from build123d import *

# Parameters (mm, degrees)
SKETCH2_W           = 35.052
SKETCH2_H           = 79.375
BOSS_EXTRUDE1_DEPTH = 22.225
SKETCH3_R           = 1.5875
BOSS_EXTRUDE2_DEPTH = 3.175
BOSS_EXTRUDE4_DEPTH = 22.225
FILLET2_R           = 3.175
BOSS_EXTRUDE5_DEPTH = 0.00254
BOSS_EXTRUDE6_START = 0.00254
BOSS_EXTRUDE6_DEPTH = 0.00254
BOSS_EXTRUDE7_DEPTH = 6.35
SKETCH8_R           = 7.441189758
SKETCH8_R_2         = 3.175
CUT_EXTRUDE2_DEPTH  = 1.5875
FILLET3_R           = 1.5875
FILLET5_R           = 1.5875
SKETCH9_R           = 4.1275
CUT_EXTRUDE3_DEPTH  = 6.858
SKETCH10_R          = 4.1275
CUT_EXTRUDE4_DEPTH  = 6.858
SKETCH11_R          = 1.5875
CUT_EXTRUDE5_DEPTH  = 91.861200127


with BuildPart() as part:
    # Sketch2 → Boss-Extrude1 (new body)
    with BuildSketch(Plane.XY):
        with Locations((17.526, 39.6875)):
            Rectangle(SKETCH2_W, SKETCH2_H)
    extrude(amount=BOSS_EXTRUDE1_DEPTH)

    # Sketch3 → Boss-Extrude2 (add)
    with BuildSketch(Plane(origin=(35.052, 0, 0), x_dir=(0, 0, -1), z_dir=(1, 0, 0))):
        with Locations(Location((-11.1125, 6.985, 0), (0, 0, 180))):
            Circle(SKETCH3_R)
    extrude(amount=BOSS_EXTRUDE2_DEPTH)

    # Sketch4 → Boss-Extrude4 (add)
    with BuildSketch(Plane.XY.offset(22.225)):
        Polygon((30.48, -3.81), (30.48, 0), (29.21, 0), (3.81, 0), (3.81, -29.21), (35.052, -29.21), (35.052, -9.836099718), align=None)
    extrude(amount=-BOSS_EXTRUDE4_DEPTH)

    # Fillet2
    fillet2_edges = [part.edges().sort_by_distance(p)[0] for p in [
        (30.48, -3.81, 11.1125),
        (35.052, -9.836099718, 11.1125),
        (35.052, -29.21, 11.1125),
        (3.81, -29.21, 11.1125),
    ]]
    fillet(fillet2_edges, radius=FILLET2_R)

    # Sketch5 → Boss-Extrude5 (add)
    with BuildSketch(Plane.XY.offset(22.225)):
        with BuildLine():
            Line((3.81, 0), (30.48, 0))
            Line((30.48, 0), (30.48, -2.741877551))
            ThreePointArc((30.48, -2.741877551), (30.64572555, -3.754247187), (31.125601437, -4.660931461))
            Line((31.125601437, -4.660931461), (34.406398563, -8.985168257))
            ThreePointArc((34.406398563, -8.985168257), (34.88627445, -9.891852531), (35.052, -10.904222168))
            Line((35.052, -10.904222168), (35.052, -26.035))
            ThreePointArc((35.052, -26.035), (34.12206403, -28.28006403), (31.877, -29.21))
            Line((31.877, -29.21), (6.985, -29.21))
            ThreePointArc((6.985, -29.21), (4.73993597, -28.28006403), (3.81, -26.035))
            Line((3.81, -26.035), (3.81, 0))
        make_face()
    extrude(amount=BOSS_EXTRUDE5_DEPTH)

    # Sketch6 → Boss-Extrude6 (add)
    with BuildSketch(Plane(origin=(0, 0, 0), x_dir=(-1, 0, 0), z_dir=(0, 0, -1)).offset(BOSS_EXTRUDE6_START)):
        with BuildLine():
            Line((-30.48, 0), (-3.81, 0))
            Line((-3.81, 0), (-3.81, -26.035))
            ThreePointArc((-3.81, -26.035), (-4.73993597, -28.28006403), (-6.985, -29.21))
            Line((-6.985, -29.21), (-31.877, -29.21))
            ThreePointArc((-31.877, -29.21), (-34.12206403, -28.28006403), (-35.052, -26.035))
            Line((-35.052, -26.035), (-35.052, -10.904222168))
            ThreePointArc((-35.052, -10.904222168), (-34.88627445, -9.891852531), (-34.406398563, -8.985168257))
            Line((-34.406398563, -8.985168257), (-31.125601437, -4.660931461))
            ThreePointArc((-31.125601437, -4.660931461), (-30.64572555, -3.754247187), (-30.48, -2.741877551))
            Line((-30.48, -2.741877551), (-30.48, 0))
        make_face()
    extrude(amount=-BOSS_EXTRUDE6_DEPTH)

    # Sketch7 → Boss-Extrude7 (add)
    with BuildSketch(Plane.XZ.offset(29.21)):
        Polygon((17.890627537, 15.85327897), (15.398252537, 14.042462536), (14.44625, 11.1125), (15.398252537, 8.182537464), (17.890627537, 6.37172103), (20.971372463, 6.37172103), (23.463747463, 8.182537464), (24.41575, 11.1125), (23.463747463, 14.042462536), (20.971372463, 15.85327897), align=None)
    extrude(amount=BOSS_EXTRUDE7_DEPTH)

    # Sketch8 → Cut-Extrude2 (cut)
    # profile 1 of 2: a face of its own
    with BuildSketch(Plane.XZ.offset(29.21)):
        with Locations((19.431, 11.1125)):
            Circle(SKETCH8_R)
        Polygon((14.44625, 11.1125), (15.398252537, 14.042462536), (17.890627537, 15.85327897), (20.971372463, 15.85327897), (23.463747463, 14.042462536), (24.41575, 11.1125), (23.463747463, 8.182537464), (20.971372463, 6.37172103), (17.890627537, 6.37172103), (15.398252537, 8.182537464), align=None, mode=Mode.SUBTRACT)
    # profile 2 of 2: a face of its own
    with BuildSketch(Plane.XZ.offset(29.21)):
        Polygon((15.398252537, 14.042462536), (17.890627537, 15.85327897), (20.971372463, 15.85327897), (23.463747463, 14.042462536), (24.41575, 11.1125), (23.463747463, 8.182537464), (20.971372463, 6.37172103), (17.890627537, 6.37172103), (15.398252537, 8.182537464), (14.44625, 11.1125), align=None)
        with Locations(Location((19.431, 11.1125, 0), (0, 0, 270))):
            Circle(SKETCH8_R_2, mode=Mode.SUBTRACT)
    extrude(amount=CUT_EXTRUDE2_DEPTH, mode=Mode.SUBTRACT)

    # Fillet3
    fillet3_edges = [part.edges().sort_by_distance(p)[0] for p in [
        (0, 79.375, 11.1125),
        (35.052, 79.375, 11.1125),
        (35.052, 0, 11.1125),
        (0, 0, 11.1125),
    ]]
    fillet(fillet3_edges, radius=FILLET3_R)

    # Fillet5
    # the kernel refuses this fillet: 1.5875 mm, written as the material it takes off along each edge
    with BuildSketch(Plane(origin=(30.48, -2.741877551, -0.00254), x_dir=(0, 0, 1), z_dir=(0, 1, 0)), Plane(origin=(30.48, 0, 22.22754), x_dir=(0, 0, -1), z_dir=(0, -1, 0))) as fillet5_piece_1:
        with BuildLine():
            CenterArc((FILLET5_R, -FILLET5_R), FILLET5_R, 90, 90)
            Line((0, -FILLET5_R), (0, 0))
            Line((0, 0), (FILLET5_R, 0))
        make_face()
    extrude(amount=2.741877551, mode=Mode.SUBTRACT)
    with BuildSketch(Plane(origin=(33.655, -2.741877551, -0.00254), x_dir=(-0.7966609646289196, -0.6044264284729114, 0), z_dir=(0.6044264284729114, -0.7966609646289196, 0))) as fillet5_piece_2:
        with BuildLine():
            CenterArc((3.175 + FILLET5_R, -FILLET5_R), FILLET5_R, 90, 90)
            Line((3.175, -FILLET5_R), (3.175, 0))
            Line((3.175, 0), (3.175 + FILLET5_R, 0))
        make_face()
    revolve(axis=Axis((33.655, -2.741877551, -0.00254), (0, 0, -1)), revolution_arc=37.18757939, mode=Mode.SUBTRACT)
    with BuildSketch(Plane(origin=(34.406398563, -8.985168257, -0.00254), x_dir=(-0.796660964628914, -0.6044264284729185, 0), z_dir=(-0.6044264284729186, 0.7966609646289141, 0)), Plane(origin=(31.125601437, -4.660931461, 22.22754), x_dir=(-0.7966609646289139, -0.6044264284729186, 0), z_dir=(0.6044264284729186, -0.796660964628914, 0))) as fillet5_piece_3:
        with BuildLine():
            CenterArc((FILLET5_R, FILLET5_R), FILLET5_R, 180, 90)
            Line((0, FILLET5_R), (0, 0))
            Line((0, 0), (FILLET5_R, 0))
        make_face()
    extrude(amount=5.427951146, mode=Mode.SUBTRACT)
    with BuildSketch(Plane(origin=(31.877, -10.904222168, -0.00254), x_dir=(1, 0, 0), z_dir=(0, -1, 0))) as fillet5_piece_4:
        with BuildLine():
            CenterArc((3.175 - FILLET5_R, FILLET5_R), FILLET5_R, 270, 90)
            Line((3.175, FILLET5_R), (3.175, 0))
            Line((3.175, 0), (3.175 - FILLET5_R, 0))
        make_face()
    revolve(axis=Axis((31.877, -10.904222168, -0.00254), (0, 0, 1)), revolution_arc=37.18757939, mode=Mode.SUBTRACT)
    with BuildSketch(Plane(origin=(35.052, -26.035, -0.00254), x_dir=(-1, 0, 0), z_dir=(0, 1, 0)), Plane(origin=(35.052, -10.904222168, 22.22754), x_dir=(-1, 0, 0), z_dir=(0, -1, 0))) as fillet5_piece_5:
        with BuildLine():
            CenterArc((FILLET5_R, FILLET5_R), FILLET5_R, 180, 90)
            Line((0, FILLET5_R), (0, 0))
            Line((0, 0), (FILLET5_R, 0))
        make_face()
    extrude(amount=15.130777832, mode=Mode.SUBTRACT)
    with BuildSketch(Plane(origin=(31.877, -26.035, -0.00254), x_dir=(0, -1, 0), z_dir=(-1, 0, 0))) as fillet5_piece_6:
        with BuildLine():
            CenterArc((3.175 - FILLET5_R, FILLET5_R), FILLET5_R, 270, 90)
            Line((3.175, FILLET5_R), (3.175, 0))
            Line((3.175, 0), (3.175 - FILLET5_R, 0))
        make_face()
    revolve(axis=Axis((31.877, -26.035, -0.00254), (0, 0, 1)), revolution_arc=90, mode=Mode.SUBTRACT)
    with BuildSketch(Plane(origin=(6.985, -29.21, -0.00254), x_dir=(0, 1, 0), z_dir=(1, 0, 0)), Plane(origin=(31.877, -29.21, 22.22754), x_dir=(0, 1, 0), z_dir=(-1, 0, 0))) as fillet5_piece_7:
        with BuildLine():
            CenterArc((FILLET5_R, FILLET5_R), FILLET5_R, 180, 90)
            Line((0, FILLET5_R), (0, 0))
            Line((0, 0), (FILLET5_R, 0))
        make_face()
    extrude(amount=24.892, mode=Mode.SUBTRACT)
    with BuildSketch(Plane(origin=(6.985, -26.035, -0.00254), x_dir=(-1, 0, 0), z_dir=(0, 1, 0))) as fillet5_piece_8:
        with BuildLine():
            CenterArc((3.175 - FILLET5_R, FILLET5_R), FILLET5_R, 270, 90)
            Line((3.175, FILLET5_R), (3.175, 0))
            Line((3.175, 0), (3.175 - FILLET5_R, 0))
        make_face()
    revolve(axis=Axis((6.985, -26.035, -0.00254), (0, 0, 1)), revolution_arc=90, mode=Mode.SUBTRACT)
    with BuildSketch(Plane(origin=(3.81, 0, -0.00254), x_dir=(0, 0, 1), z_dir=(0, -1, 0)), Plane(origin=(3.81, -26.035, 22.22754), x_dir=(0, 0, -1), z_dir=(0, 1, 0))) as fillet5_piece_9:
        with BuildLine():
            CenterArc((FILLET5_R, -FILLET5_R), FILLET5_R, 90, 90)
            Line((0, -FILLET5_R), (0, 0))
            Line((0, 0), (FILLET5_R, 0))
        make_face()
    extrude(amount=26.035, mode=Mode.SUBTRACT)
    with BuildSketch(Plane(origin=(6.985, -26.035, 22.22754), x_dir=(0, -1, 0), z_dir=(1, 0, 0))) as fillet5_piece_10:
        with BuildLine():
            CenterArc((3.175 - FILLET5_R, FILLET5_R), FILLET5_R, 270, 90)
            Line((3.175, FILLET5_R), (3.175, 0))
            Line((3.175, 0), (3.175 - FILLET5_R, 0))
        make_face()
    revolve(axis=Axis((6.985, -26.035, 22.22754), (0, 0, -1)), revolution_arc=90, mode=Mode.SUBTRACT)
    with BuildSketch(Plane(origin=(31.877, -26.035, 22.22754), x_dir=(1, 0, 0), z_dir=(0, 1, 0))) as fillet5_piece_11:
        with BuildLine():
            CenterArc((3.175 - FILLET5_R, FILLET5_R), FILLET5_R, 270, 90)
            Line((3.175, FILLET5_R), (3.175, 0))
            Line((3.175, 0), (3.175 - FILLET5_R, 0))
        make_face()
    revolve(axis=Axis((31.877, -26.035, 22.22754), (0, 0, -1)), revolution_arc=90, mode=Mode.SUBTRACT)
    with BuildSketch(Plane(origin=(31.877, -10.904222168, 22.22754), x_dir=(0.7966609646289129, 0.6044264284729202, 0), z_dir=(-0.6044264284729202, 0.7966609646289129, 0))) as fillet5_piece_12:
        with BuildLine():
            CenterArc((3.175 - FILLET5_R, FILLET5_R), FILLET5_R, 270, 90)
            Line((3.175, FILLET5_R), (3.175, 0))
            Line((3.175, 0), (3.175 - FILLET5_R, 0))
        make_face()
    revolve(axis=Axis((31.877, -10.904222168, 22.22754), (0, 0, -1)), revolution_arc=37.18757939, mode=Mode.SUBTRACT)
    with BuildSketch(Plane(origin=(33.655, -2.741877551, 22.22754), x_dir=(-1, 0, 0), z_dir=(0, 1, 0))) as fillet5_piece_13:
        with BuildLine():
            CenterArc((3.175 + FILLET5_R, -FILLET5_R), FILLET5_R, 90, 90)
            Line((3.175, -FILLET5_R), (3.175, 0))
            Line((3.175, 0), (3.175 + FILLET5_R, 0))
        make_face()
    revolve(axis=Axis((33.655, -2.741877551, 22.22754), (0, 0, 1)), revolution_arc=37.18757939, mode=Mode.SUBTRACT)

    # Sketch9 → Cut-Extrude3 (cut)
    with BuildSketch(Plane(origin=(35.052, 0, 0), x_dir=(0, 0, -1), z_dir=(1, 0, 0))):
        with Locations((-11.1125, 55.88)):
            Circle(SKETCH9_R)
        with Locations((-11.1125, 36.83)):
            Circle(SKETCH9_R)
    extrude(amount=-CUT_EXTRUDE3_DEPTH, mode=Mode.SUBTRACT)

    # Sketch10 → Cut-Extrude4 (cut)
    with BuildSketch(Plane.ZY):
        with Locations((11.1125, 65.7225)):
            Circle(SKETCH10_R)
        with Locations((11.1125, 46.6725)):
            Circle(SKETCH10_R)
        with Locations((11.1125, 27.6225)):
            Circle(SKETCH10_R)
    extrude(amount=-CUT_EXTRUDE4_DEPTH, mode=Mode.SUBTRACT)

    # Sketch11 → Cut-Extrude5 (cut, through all)
    with BuildSketch(Plane.XY.offset(22.225)):
        with Locations((4.7625, 56.1975)):
            Circle(SKETCH11_R)
        with Locations((4.7625, 37.1475)):
            Circle(SKETCH11_R)
    extrude(amount=-CUT_EXTRUDE5_DEPTH, mode=Mode.SUBTRACT)


solid = part.part
Work out the finished part from the listing and answer in its coordinate system (mm). A direction names the side the tool comes from. Round coordinates to 2 decimals unless told otherwise and drop trailing zeros. Write each loop counter-clockwise with the first axis right and the second up, starting at its lowest first coordinate (ties: lowest second). Pieces come first, ordered by that corner, then holes.
1) A cutting plane is placed at B-B (y = 29). Give the vertices of the cut face in (x, z) (3 decimals).
2) Given pin 1 Ø12 at (x, y) = (26.5, 44) entering from +Z (3 decimals); pin 2 Ø10.5 at (y, z) = (55.88, 11.11) entering from +X; pin 3 Ø2.5 at (y, z) = (66, 9.5) entering from -X, each flat-ended and moving along its own axis, determine where each tip first touches the part or whether it passes through.
3) The mould has two halves that part along X. Classify faces 1 (the cylindrical face through (3.381, 23.593, 10.218)), 2 (the cylindrical face through (5.5, 54.79, 11.27)), 3 (the cylindrical face through (30.64, -3.74, 10.98)): pulls with the +X half, pulls with the -X half, needs draft (parallel to the pull), parting line crosses it, or undercut.
4) A tool of negligible diameter and unlimited length cuts with its end or side. For faces 4 (the flat face through (14.93, -33.15, 12.6)), 5 (the flat face through (6.858, 28, 11)), 6 (the cylindrical face through (34.891, -9.906, 10.979)), 7 (the flat face through (28.194, 37, 11)), from which of +Z, -Z, +X, -X, +Y, -Y can it reach the whole face along a straight path? Write none if from no direction.
5) Straight lines are drawn through the part: line 1 (Y direction, x = 22.5, z = 8.5) (1 decimal); line 2 (Y direction, x = 4.5, z = 20.25) (3 decimals); line 3 (Y direction, x = 28.5, z = 1.5) (3 decimals). For each, find the intervals that lie inside material, in ascending order.
6) A cutting plane is placed at A-A (y = -22). Give the vertices of the cut face in (x, z) (1 decimal).
Completed:
1. outline: (0, 0) - (35.052, 0) - (35.052, 22.225) - (0, 22.225) - (0, 15.003) - (6.858, 15.003) - (6.858, 7.222) - (0, 7.222) - close
2. pin 1: stops at z = 22.225
2. pin 2: stops at x = 35.05
2. pin 3: stops at x = 6.86
3. face 1: needs draft
3. face 2: undercut
3. face 3: pulls with the +X half
4. face 4: +Z, -X, -Y
4. face 5: -X
4. face 6: +Z, -Z, +X
4. face 7: +X
5. line 1: y = -35.6 to -30.8, -29.2 to 79.4
5. line 2: y = -28.011 to 35.582, 38.713 to 54.632, 57.763 to 79.375
5. line 3: y = -29.208 to 79.375
6. outline: (3.8, 1.6) arc R1.6 ccw to (5.4, 0) - (33.5, 0) arc R1.6 ccw to (35.1, 1.6) - (35.1, 20.6) arc R1.6 ccw to (33.5, 22.2) - (5.4, 22.2) arc R1.6 ccw to (3.8, 20.6) - close
